Geometry check sheet. Reference: drawing and pictorial views, mm from the part's lowest x, y, z. Round coordinates to 2 decimals unless told otherwise and drop trailing zeros. Write each loop counter-clockwise with the first axis right and the second up, starting at its lowest first coordinate (ties: lowest second). Pieces come first, ordered by that corner, then holes. Notation, with made-up numbers: (54.25, -4.5) -> (102.25, -4.5) arc R32 ccw to (102.25, 25.5) -> close; hole circle Ø5 at (16, 0.5). An arc over 180 degrees is marked (long way). Answer as a JSON object with one key per item and string values. Group by question number.
(1) Sectioned sample at B-B on z = 1.75. Record the cut outline in (x, y), and give its area (3 significant figures).
(2) Sectioned sample at D-D on x = 9.75. Record the cut outline in (y, z).
(3) Gauge pin test, flat end, axial feed: pin 1 Ø3 at (x, z) = (6.06, 3.225) entering from -Y. Record the tip position at first contact, or that the pin passes through.
(4) Sectioned sample at C-C on y = 0.2. Record the cut outline in (x, z) (3 decimals), and give its area (3 significant figures).
(5) Draft check along X on the marked faces 1, 2 and 3. Enter one of: released by +X, released by -X, zero draft, split by the parting line, or undercut.
(6) Sectioned sample at A-A on x = 6.06. Record the cut outline in (y, z) (3 decimals).
(7) Scan lines: L1, parallel to Z at x = 6.06, y = 0.45 (3 decimals); L2, parallel to X at y = 0.35, z = 2.75; L3, parallel to Z at x = 6.5, y = 0.6. Record each from-to range of solid material in increasing order. Write a range as from..to.
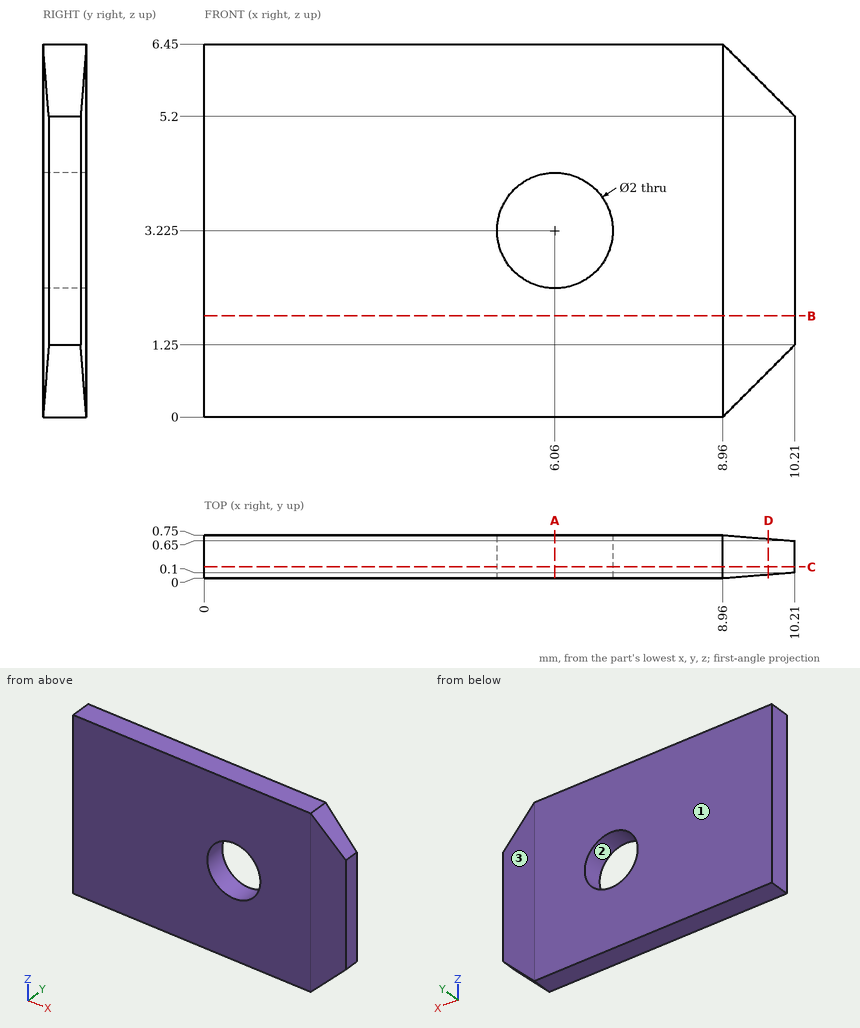
Computed values:
{
 "1": {"outline": "(0, 0) -> (8.96, 0) -> (10.21, 0.1) -> (10.21, 0.65) -> (8.96, 0.75) -> (0, 0.75) -> close", "area": "7.53 mm2"},
 "2": {"outline": "(0.06, 0.79) -> (0.69, 0.79) -> (0.69, 5.66) -> (0.06, 5.66) -> close"},
 "3": {"pin 1": "y = 0"},
 "4": {"outline": "(0, 0) -> (8.96, 0) -> (10.21, 1.25) -> (10.21, 5.2) -> (8.96, 6.45) -> (0, 6.45) -> close; hole circle Ø2 at (6.06, 3.225)", "area": "61.2 mm2"},
 "5": {"face 1": "zero draft", "face 2": "undercut", "face 3": "released by +X"},
 "6": {"outline": "(0, 0) -> (0.75, 0) -> (0.75, 2.225) -> (0, 2.225) -> close; (0, 4.225) -> (0.75, 4.225) -> (0.75, 6.45) -> (0, 6.45) -> close"},
 "7": {"L1": "0..2.225, 4.225..6.45", "L2": "0..5.18, 6.94..10.21", "L3": "0..2.33, 4.12..6.45"}
}
